Source: CAD feature listing. Evaluate the final solid. Frame: model axes, mm. A direction names the side the tool comes from. Round coordinates to 2 decimals unless told otherwise and drop trailing zeros. Write each loop counter-clockwise with the first axis right and the second up, starting at its lowest first coordinate (ties: lowest second). Pieces come first, ordered by that corner, then holes.
from build123d import *

# Parameters (mm, degrees)
SKETCH1_R           = 2
SKETCH1_R_2         = 3.175
BOSS_EXTRUDE1_DEPTH = 6.35


with BuildPart() as part:
    # Sketch1 → Boss-Extrude1 (new body)
    with BuildSketch(Plane(origin=(0, 0, 0), x_dir=(0, 0, -1), z_dir=(1, 0, 0))):
        Polygon((28.575, -22.225), (28.575, -28.575), (34.925, -28.575), (34.925, -22.225), (44.45, -22.225), (44.45, -15.875), (38.1, -15.875), (38.1, -9.8806), (44.45, -9.8806), (44.45, 38.1), (38.1, 38.1), (38.1, 44.0944), (44.45, 44.0944), (44.45, 47.625), (-44.45, 47.625), (-44.45, 44.0944), (-38.1, 44.0944), (-38.1, 38.1), (-44.45, 38.1), (-44.45, 22.225), (-44.45, -9.8806), (-38.1, -9.8806), (-38.1, -15.875), (-44.45, -15.875), (-44.45, -22.225), (-34.925, -22.225), (-34.925, -28.575), (-28.575, -28.575), (-28.575, -22.225), (-6.35, -22.225), (-6.35, -28.575), (6.35, -28.575), (6.35, -22.225), align=None)
        with Locations((25.309068, -7.724902)):
            Circle(SKETCH1_R, mode=Mode.SUBTRACT)
        Circle(SKETCH1_R_2, mode=Mode.SUBTRACT)
    extrude(amount=BOSS_EXTRUDE1_DEPTH)


solid = part.part
1) Material intervals for line 1 (Z direction, x = 4.5, y = -24.5) (3 decimals); line 2 (Y direction, x = 4.25, z = -39.5) (3 decimals); line 3 (Z direction, x = 4.75, y = -8), sorted ascending.
Taken from the geometry:
line 1: z = -34.925 to -28.575, -6.35 to 6.35, 28.575 to 34.925
line 2: y = -22.225 to -15.875, -9.881 to 38.1, 44.094 to 47.625
line 3: z = -44.45 to -27.29, -23.33 to 44.45
2) Contact query for flat-ended pins moving along their axis: P1, Ø3, axis at x = 2, z = 41, coming from the -Y side (3 decimals); P2, Ø3, axis at x = 2, y = -24.5, coming from the +Z side (3 decimals); P3, Ø3, axis at x = 3, y = -13, coming from the -Z side. Output: stop coordinate, or through.
Taken from the geometry:
P1: stops at y = -22.225
P2: stops at z = 34.925
P3: stops at z = -38.1
3) Section query D-D on z = -14. Return the cut outline in (x, y) (3 decimals), then the cut area to 3 significant figures.
Taken from the geometry:
outline: (0, -22.225) - (6.35, -22.225) - (6.35, 47.625) - (0, 47.625) - close
area: 444 mm2
4) Section query C-C on x = 4.5. State how many separate pieces and enclosed holes the cut face has, then the cut area to 3 significant figures.
Taken from the geometry:
separate pieces: 1
enclosed holes: 2
area: 6,170 mm2
5) Section query B-B on z = 0. Return the cut outline in (x, y) (3 decimals), then the cut area to 3 significant figures.
Taken from the geometry:
outline: (0, -28.575) - (6.35, -28.575) - (6.35, -3.175) - (0, -3.175) - close; (0, 3.175) - (6.35, 3.175) - (6.35, 47.625) - (0, 47.625) - close
area: 444 mm2
6) Section query A-A on y = 0. Return the cut outline in (x, z) (3 decimals).
Taken from the geometry:
outline: (0, -44.45) - (6.35, -44.45) - (6.35, -3.175) - (0, -3.175) - close; (0, 3.175) - (6.35, 3.175) - (6.35, 44.45) - (0, 44.45) - close
7) Reachability of faces 1 (the face through (3, -25, 6.35)), 2 (the face through (3, 44.094, -41)), 3 (the face through (3, -13, 38.1)) from +Z, -Z, +X, -X, +Y, -Y: full face, straight path, thin tool, end or side. Return the list, or none.
Taken from the geometry:
face 1: +X, -X, -Y
face 2: -Z, +X, -X
face 3: +Z, +X, -X
8) Pull-direction query (Z, two-part tool) for faces 4 (the face through (3, -9.881, -41)), 5 (the face through (3.131, -8.491, -27.157)), 6 (the face through (3, 14, 44.45)); classes: released by +Z, released by -Z, zero draft, split by the parting line, or undercut.
Taken from the geometry:
face 4: zero draft
face 5: undercut
face 6: released by +Z
